Build history of the part. All positions in model axes, mm. Give positions to 0.01 mm unless a question says otherwise; leave off trailing zeros. Write each loop counter-clockwise with the first axis right and the second up, starting at its lowest first coordinate (ties: lowest second). Pieces come first, ordered by that corner, then holes. Notation, with made-up numbers: (61.5, 4.5) -> (104.5, 4.5) arc R16 ccw to (104.5, 18.5) -> close; hole circle Ø8 at (18.25, -10). An arc over 180 degrees is marked (long way). Put each result on its own line as item: value.
from build123d import *

# Parameters (mm, degrees)
SKETCH2_R           = 1.256430983
SKETCH2_R_2         = 1.905
SKETCH2_R_3         = 1.776231012
BOSS_EXTRUDE2_DEPTH = 3.175


with BuildPart() as part:
    # Sketch2 → Boss-Extrude2 (new body)
    with BuildSketch(Plane(origin=(0, 0, 0), x_dir=(1, 0, 0), z_dir=(0, 1, 0))):
        Polygon((25.4, -151.533371864), (-25.4, -151.533371864), (-25.4, -126.133371864), (-12.7, -126.133371864), (-12.7, -80.413371864), (-25.4, -80.413371864), (-68.619910987, -49.323669691), (-68.619910987, 0), (-68.619910987, 112.251832626), (-25.4, 165.193433608), (-12.7, 165.193433608), (-12.7, 200.795669484), (-25.4, 200.795669484), (-25.4, 226.195669484), (25.4, 226.195669484), (25.4, 200.795669484), (12.7, 200.795669484), (12.7, 165.193433608), (25.4, 165.193433608), (68.619910987, 112.251832626), (68.619910987, 0), (68.619910987, -49.323669691), (25.4, -80.413371864), (12.7, -80.413371864), (12.7, -126.133371864), (25.4, -126.133371864), align=None)
        with Locations(Location((-9.525, 219.845669484, 0), (0, 0, 270))):
            Circle(SKETCH2_R, mode=Mode.SUBTRACT)
        with Locations(Location((9.525, 219.845669484, 0), (0, 0, 270))):
            Circle(SKETCH2_R, mode=Mode.SUBTRACT)
        with Locations(Location((0, 207.145669484, 0), (0, 0, 270))):
            Circle(SKETCH2_R, mode=Mode.SUBTRACT)
        with Locations(Location((9.525, -145.279330516, 0), (0, 0, 270))):
            Circle(SKETCH2_R_2, mode=Mode.SUBTRACT)
        with Locations(Location((0, -132.579330516, 0), (0, 0, 270))):
            Circle(SKETCH2_R_2, mode=Mode.SUBTRACT)
        with Locations(Location((-9.525, -145.279330516, 0), (0, 0, 270))):
            Circle(SKETCH2_R_2, mode=Mode.SUBTRACT)
        with Locations(Location((-9.525, 99.829892631, 0), (0, 0, 270))):
            Circle(SKETCH2_R_3, mode=Mode.SUBTRACT)
        with Locations(Location((9.525, 99.829892631, 0), (0, 0, 270))):
            Circle(SKETCH2_R_3, mode=Mode.SUBTRACT)
    extrude(amount=BOSS_EXTRUDE2_DEPTH)


solid = part.part
1) Slice it at B-B (y = 1). Give the number of separate pieces and of enclosed holes in the cut face, plus the area to 3 significant figures.
Filled sheet:
separate pieces: 1
enclosed holes: 8
area: 34,700 mm2
2) Slice it at A-A (x = -20). Write the cut outline in (y, z) (3 decimals).
Filled sheet:
outline: (0, -226.196) -> (3.175, -226.196) -> (3.175, -200.796) -> (0, -200.796) -> close; (0, -165.193) -> (3.175, -165.193) -> (3.175, 80.413) -> (0, 80.413) -> close; (0, 126.133) -> (3.175, 126.133) -> (3.175, 151.533) -> (0, 151.533) -> close
3) Wall check: L1, parallel to Z at x = 18.5, y = 2.8; L2, parallel to Z at x = 8, y = 2.35; L3, parallel to X at y = 2, z = -186. Give the ranges that are in metal, low to high.
Filled sheet:
L1: -226.2 to -200.8, -165.19 to 80.41, 126.13 to 151.53
L2: -226.2 to -100.74, -98.92 to 144.14, 146.42 to 151.53
L3: -12.7 to 12.7
4) Slice it at C-C (z = -132). Write the cut outline in (x, y) (3 decimals).
Filled sheet:
outline: (-52.498, 0) -> (52.498, 0) -> (52.498, 3.175) -> (-52.498, 3.175) -> close
5) Pin check, flat tips, straight feed: pin 1 (1.5 mm diameter, centred on y = 2, z = 108, fed in from -X); pin 2 (1.6 mm diameter, centred on y = 1.5, z = -181.5, fed in from +X); pin 3 (2 mm diameter, centred on x = -9.52, z = -99.83, fed in from +Y); pin 4 (1.6 mm diameter, centred on y = 1, z = -216, fed in from +X). Stop position of each tip, or through.
Filled sheet:
pin 1: x = -12.7
pin 2: x = 12.7
pin 3: through
pin 4: x = 25.4
6) Slice it at D-D (x = -49.5). Write the cut outline in (y, z) (3 decimals), plus the area to 3 significant figures.
Filled sheet:
outline: (0, -135.672) -> (3.175, -135.672) -> (3.175, 63.077) -> (0, 63.077) -> close
area: 631 mm2
